Here's how the part is built. I have some questions about the finished solid (model axes, mm). A direction names the side the tool comes from. Round coordinates to 2 decimals unless told otherwise and drop trailing zeros. Loops run counter-clockwise (first coordinate to the right, second up) from the corner with the lowest first, then second, coordinate; pieces in that order, holes last. Notation, with made-up numbers: M -2.75,84 L 38.25,84 A24 cw 38.25,112 Z; hole C 3,39 d8. An arc over 180 degrees is marked long. One line per question, with ' | ' between items. Start each with the question number.
Autodesk Inventor part; units mm, degrees
ref_plane "YZ Plane" through (0, 0, 0) normal (1, 0, 0) x (0, 1, 0)
ref_plane "XZ Plane" through (0, 0, 0) normal (0, 1, 0) x (-1, 0, 0)
ref_plane "XY Plane" through (0, 0, 0) normal (0, 0, 1) x (1, 0, 0)
sketch "Sketch1" plane through (0, 0, 0) normal (0, 0, 1) x (1, 0, 0)
  line L0 (-21.15, 19.15) -> (-21.15, -19.15)
  line L1 (21.15, -19.15) -> (21.15, 19.15)
  line L2 (19.15, 21.15) -> (-19.15, 21.15)
  line L3 (-19.15, -21.15) -> (19.15, -21.15)
  line L4 (159.3629, -5.0795) -> (159.3629, 4.9205)
  line L5 (159.3629, -5.0795) -> (159.3629, 4.9205)
  line L6 (159.3629, 4.9205) -> (138.2729, 4.9205)
  line L7 (138.2729, -5.0795) -> (159.3629, -5.0795)
  circle A0 centre (-15.5, -15.5) radius 2.55
  circle A1 centre (15.5, 15.5) radius 2.55
  circle A2 centre (-15.5, 15.5) radius 2.55
  circle A3 centre (15.5, -15.5) radius 2.55
  line L8 (-21.15, -19.15) -> (-21.15, 19.15)
  line L9 (-19.15, 21.15) -> (19.15, 21.15)
  line L10 (21.15, 19.15) -> (21.15, -19.15)
  line L11 (19.15, -21.15) -> (-19.15, -21.15)
  arc A4 (-21.15, -19.15) -> (-19.15, -21.15) centre (-19.15, -19.15) ccw
  arc A5 (-19.15, 21.15) -> (-21.15, 19.15) centre (-19.15, 19.15) ccw
  arc A6 (21.15, 19.15) -> (19.15, 21.15) centre (19.15, 19.15) ccw
  arc A7 (19.15, -21.15) -> (21.15, -19.15) centre (19.15, -19.15) ccw
  circle A8 centre (-15.5, -15.5) radius 2.55
  circle A9 centre (-15.5, 15.5) radius 2.55
  circle A10 centre (15.5, 15.5) radius 2.55
  circle A11 centre (15.5, -15.5) radius 2.55
  line L12 (159.3629, -5.0795) -> (21.15, -5.0795)
  line L13 (159.3629, -5.0795) -> (159.3629, 4.9205)
  line L14 (159.3629, 4.9205) -> (21.15, 4.9205)
  point P0 (0, 0)
  dimension "d0" = 2
sketch "Sketch2" plane through (159.3629, -5.0795, 0) normal (1, 0, 0) x (0, 0, -1)
  line L0 (91.2, 0) -> (91.2, 10)
  line L1 (65, 0) -> (65, 10)
  circle A0 centre (78.1, 5) radius 2.75
  line L2 (-5, 10) -> (-5, 0)
  line L3 (0, 10) -> (-5, 10)
  line L4 (0, 0) -> (-5, 0)
  line L5 (-5, 10) -> (91.2, 10)
  line L6 (91.2, 10) -> (91.2, 0)
  line L7 (91.2, 0) -> (-5, 0)
  line L8 (-5, 0) -> (-5, 10)
  circle A1 centre (78.1, 5) radius 2.75
  point P0 (0, 5.0795)
extrude "Plate1" add sketch "Sketch1" along normal blind 5
sheet face with bend "Face2" sketch "Sketch2" thickness 5 toward (1, 0, 0) bend radius 5
bend "Bend1"
equation "\"d1\" = Thickness"
equation "\"d2\" = BendRadius"
equation "\"d3\" = BendReliefWidth"
equation "\"d5\" = MinimumRemnant"
equation "\"d4\" = BendReliefDepth"
equation "\"d6\" = TransitionRadius"
equation "\"BendRadius\" = Thickness"
equation "\"BendReliefWidth\" = Thickness"
equation "\"BendReliefDepth\" = 0.5 * Thickness"
equation "\"TransitionRadius\" = BendRadius"
equation "\"JacobiRadiusSize\" = BendRadius"
equation "\"GapSize\" = Thickness"
properties part number "corredera"
1) We'd pull the mould along Y, two halves only. Please class faces 6 (the face through (-17.524, 17.052, 2.465)), 7 (the face through (125, 4.92, 3)), 8 (the face through (13.476, -13.948, 2.465)), 9 (the face through (26, 0, 5)): pulls with the +Y half, pulls with the -Y half, needs draft (parallel to the pull), parting line crosses it, or undercut.
2) Imagine slicing it at B-B (y = -15.5). Write out the boundary of the cut face in (x, z), then the cut area to 4 significant figures.
3) Imagine slicing it at A-A (z = -78.1). Write out the boundary of the cut face in (x, y).
4) For faces 1 (the face through (0, 21.15, 2)), 2 (the face through (21.15, 12, 2)), 3 (the face through (13.476, 17.052, 2.465)), 4 (the face through (159.363, 0, -47)), 5 (the face through (21.15, -12, 2)), which set-ups out of +Z, -Z, +X, -X, +Y, -Y let a thin tool reach every point of the face, with its end or its side?
5) I'm going to push flat-ended pins straight in: pin 1 Ø1.5 at (y, z) = (10, 3.5) entering from +X; pin 2 Ø6.5 at (x, y) = (15.5, -15.5) entering from -Z; pin 3 Ø11 at (y, z) = (-2, -61.5) entering from -X. Where does each tip first touch, or does it pass through?
6) Please list where these lines run through material, in increasing order: L1, parallel to Y at x = 15.5, z = 2.8; L2, parallel to X at y = 15, z = 1; L3, parallel to X at y = 4, z = -60. Write a range as from..to.
7) Imagine slicing it at D-D (x = 7). Write out the boundary of the cut face in (y, z).
Results are:
1) face 6: undercut | face 7: pulls with the +Y half | face 8: undercut | face 9: needs draft
2) outline: M -21.15,0 L -18.05,0 L -18.05,5 L -21.15,5 Z; M -12.95,0 L 12.95,0 L 12.95,5 L -12.95,5 Z; M 18.05,0 L 21.15,0 L 21.15,5 L 18.05,5 Z | area: 160.5 mm²
3) outline: M 159.36,-5.08 L 164.36,-5.08 L 164.36,-2.83 L 159.36,-2.83 Z; M 159.36,2.67 L 164.36,2.67 L 164.36,4.92 L 159.36,4.92 Z
4) face 1: +Z, -Z, +X, -X, +Y | face 2: +Z, -Z, +X, +Y | face 3: +Z, -Z | face 4: -Z, -X, +Y, -Y | face 5: +Z, -Z, +X, -Y
5) pin 1: x = 21.15 | pin 2: z = 0 | pin 3: x = 159.36
6) L1: -21.15..-18.05, -12.95..12.95, 18.05..21.15 | L2: -21.15..-18, -13..13, 18..21.15 | L3: 159.36..164.36
7) outline: M -21.15,0 L 21.15,0 L 21.15,5 L -21.15,5 Z
